Part model, mm, in its own coordinate system. A direction names the side the tool comes from. Coordinates: 2 decimals unless noted, no trailing zeros. Loops run counter-clockwise (first coordinate to the right, second up) from the corner with the lowest first, then second, coordinate; pieces in that order, holes last. Notation, with made-up numbers: M -23.75,-32 L 0.25,-32 A26 cw 0.25,-11 Z; hole C 44.5,17.5 d3. An arc over 180 degrees is marked long. Answer as CSV lines item,"result". Start each with the question number.
Autodesk Inventor part; units mm, degrees
ref_plane "YZ Plane" through (0, 0, 0) normal (1, 0, 0) x (0, 1, 0)
ref_plane "XZ Plane" through (0, 0, 0) normal (0, 1, 0) x (-1, 0, 0)
ref_plane "XY Plane" through (0, 0, 0) normal (0, 0, 1) x (1, 0, 0)
sketch "Sketch1" plane through (0, 0, 0) normal (0, 0, 1) x (1, 0, 0)
  line L0 (0, 0) -> (1800, 0)
  line L1 (0, 0) -> (0, -40)
  line L2 (0, -40) -> (1800, -40)
  line L3 (1800, -40) -> (1800, 0)
  dimension "d0" = 1800
  dimension "d1" = 40
extrude "Extrusion1" add sketch "Sketch1" along normal blind 40
sketch "Sketch2" plane through (0, 0, 40) normal (0, 0, 1) x (1, 0, 0)
  line L0 (0, 0) -> (0, -40)
  line L1 (1800, 0) -> (0, 0)
  line L2 (0, 0) -> (40, 0)
  line L3 (0, -40) -> (1800, -40)
  line L4 (40, -40) -> (0, -40)
  line L5 (0, -40) -> (0, 0)
  line L6 (40, 0) -> (40, -40)
  line L7 (1800, -40) -> (1800, 0)
  line L8 (1800, 0) -> (1760, 0)
  line L9 (1760, -40) -> (1800, -40)
  line L10 (1760, 0) -> (1760, -40)
  line L11 (1800, 0) -> (1800, -40)
  dimension "d5" = 40
  dimension "d6" = 40
extrude "Extrusion2" add sketch "Sketch2" along normal blind 960 contours L1 L6 L3 L0 | L1 L7 L3 L10
sketch "Sketch4" plane through (1760, -40, 40) normal (-1, 0, 0) x (0, 0, 1)
  line L0 (960, 40) -> (960, 0)
  line L1 (960, 40) -> (920, 40)
  line L2 (0, 40) -> (960, 40)
  line L3 (0, 0) -> (960, 0)
  line L4 (920, 0) -> (920, 40)
  line L5 (920, 0) -> (960, 0)
  line L6 (960, 0) -> (960, 40)
  point P0 (-40, 40)
  dimension "d9" = 40
extrude "Extrusion3" add sketch "Sketch4" along normal up to surface (1720 mm away)
sketch "Sketch5" plane through (0, -40, 0) normal (0, -1, 0) x (1, 0, 0)
  line L0 (40, 40) -> (40, 960)
  line L1 (40, 960) -> (40, 1000)
  line L2 (1800, 1000) -> (0, 1000)
  line L3 (0, 1000) -> (0, 960)
  line L4 (0, 0) -> (0, 1000)
  line L5 (40, 960) -> (0, 960)
  line L6 (0, 1000) -> (40, 1000)
  line L7 (1760, 40) -> (1760, 960)
  line L8 (1760, 960) -> (1800, 960)
  line L9 (1800, 0) -> (1800, 1000)
  line L10 (1760, 960) -> (1760, 1000)
  line L11 (1760, 1000) -> (1800, 1000)
  line L12 (1800, 1000) -> (1800, 960)
  line L13 (1760, 40) -> (40, 40)
  line L14 (1760, 40) -> (1800, 40)
  line L15 (1800, 40) -> (1800, 0)
  line L16 (1800, 0) -> (1760, 0)
  line L17 (1800, 0) -> (0, 0)
  line L18 (1760, 0) -> (1760, 40)
  line L19 (0, 40) -> (40, 40)
  line L20 (40, 0) -> (40, 40)
  line L21 (0, 40) -> (0, 0)
  line L22 (40, 0) -> (0, 0)
extrude "Extrusion4" add sketch "Sketch5" along normal blind 710 contours L20 L17 L4 L19 | L5 L3 L2 L1 | L14 L9 L16 L18 | L10 L2 L9 L8
sketch "Sketch6" plane through (1760, -40, 0) normal (-1, 0, 0) x (0, 0, 1)
  line L0 (0, 40) -> (0, -710)
  line L1 (0, -610) -> (40, -610)
  line L2 (40, 0) -> (40, -710)
  line L3 (0, -610) -> (0, -650)
  line L4 (0, -650) -> (40, -650)
  line L5 (40, -650) -> (40, -610)
  line L6 (0, 0) -> (40, 0)
  line L7 (960, 0) -> (960, -710)
  line L8 (960, -610) -> (1000, -610)
  line L9 (1000, 0) -> (1000, -710)
  line L10 (960, -650) -> (1000, -650)
  line L11 (1000, -650) -> (1000, -610)
  line L12 (960, -610) -> (960, -650)
  dimension "d14" = 40
  dimension "d15" = 650
extrude "Extrusion5" add sketch "Sketch6" along normal up to surface (1720 mm away) contours L1 L2 L4 L0 | L8 L9 L10 L7
sketch "Sketch7" plane through (0, -750, 40) normal (0, 0, 1) x (1, 0, 0)
  line L0 (40, 710) -> (40, 100)
  line L1 (40, 100) -> (0, 100)
  line L2 (0, 100) -> (0, 60)
  line L3 (40, 60) -> (40, 0)
  line L4 (0, 60) -> (40, 60)
  line L5 (40, 60) -> (40, 100)
  line L6 (1760, 60) -> (1760, 0)
  line L7 (1760, 60) -> (1800, 60)
  line L8 (1800, 710) -> (1800, 0)
  line L9 (1760, 710) -> (1760, 100)
  line L10 (1800, 100) -> (1760, 100)
  line L11 (1760, 100) -> (1760, 60)
  line L12 (0, 100) -> (0, 60)
  line L13 (0, 710) -> (0, 0)
  line L14 (1800, 100) -> (1800, 60)
  line L15 (0, 100) -> (0, 60)
  point P0 (0, 750)
extrude "Extrusion6" add sketch "Sketch7" along normal up to surface (920 mm away)
sketch "Sketch8" plane through (0, 0, 0) normal (-1, 0, 0) x (0, 0, 1)
  line L0 (40, -650) -> (960, -650)
  line L1 (902, -650) -> (902, -420)
  line L2 (902, -420) -> (722, -420)
  line L3 (722, -420) -> (722, -650)
  line L4 (960, -40) -> (960, -650)
  line L5 (722, -450) -> (902, -450)
  line L6 (722, -650) -> (902, -650)
  line L7 (764.1942, -450) -> (764.1942, -650)
  line L8 (794.1942, -450) -> (794.1942, -650)
  line L9 (826.1942, -450) -> (826.1942, -650)
  line L10 (856.1942, -450) -> (856.1942, -650)
  line L11 (872.1942, -450) -> (872.1942, -650)
  line L12 (748.1942, -450) -> (748.1942, -650)
  point P0 (0, 0)
  dimension "d20" = 230
  dimension "d21" = 58
  dimension "d22" = 180
  dimension "d23" = 30
  dimension "d24" = 30
  dimension "d25" = 30
  dimension "d26" = 32
  dimension "d27" = 16
  dimension "d28" = 16
extrude "Extrusion7" add sketch "Sketch8" against normal blind 30 contours L3 L5 L12 L0 | L3 L2 L1 L5 | L7 L5 L8 L0 | L9 L5 L10 L0 | L1 L0 L11 L5
sketch "Sketch9" plane through (1760, -690, 960) normal (0, 0, -1) x (-1, 0, 0)
  line L0 (0, 40) -> (1720, 40)
  line L1 (110, 40) -> (140, 40)
  line L2 (140, 40) -> (140, 10)
  line L3 (140, 10) -> (110, 10)
  line L4 (110, 10) -> (110, 40)
  line L5 (610, 40) -> (640, 40)
  line L6 (640, 40) -> (640, 10)
  line L7 (640, 10) -> (610, 10)
  line L8 (610, 10) -> (610, 40)
  line L9 (1080, 40) -> (1110, 40)
  line L10 (1110, 40) -> (1110, 10)
  line L11 (1110, 10) -> (1080, 10)
  line L12 (1080, 10) -> (1080, 40)
  line L13 (1580, 40) -> (1610, 40)
  line L14 (1610, 40) -> (1610, 10)
  line L15 (1610, 10) -> (1580, 10)
  line L16 (1580, 10) -> (1580, 40)
  line L17 (-40, -60) -> (-40, 690)
  line L18 (1760, 690) -> (1760, -60)
  point P0 (1610, 40)
  point P1 (1580, 40)
  point P2 (640, 40)
  point P3 (610, 40)
  dimension "d31" = 30
  dimension "d32" = 30
  dimension "d33" = 30
  dimension "d34" = 30
  dimension "d35" = 30
  dimension "d36" = 30
  dimension "d37" = 30
  dimension "d38" = 30
  dimension "d39" = 150
  dimension "d40" = 150
  dimension "d41" = 470
  dimension "d42" = 470
extrude "Extrusion8" add sketch "Sketch9" along normal up to surface (920 mm away)
sketch "Sketch24" plane through (0, -750, 0) normal (0, -1, 0) x (1, 0, 0)
  circle A0 centre (20, 20) radius 6
  line L0 (40, 40) -> (0, 40)
  line L1 (0, 40) -> (0, 0)
  point P0 (0, 20)
  dimension "d95" = 20
  dimension "d96" = 20
  dimension "d97" = 12
sketch "Sketch25" plane through (0, -750, 0) normal (0, -1, 0) x (1, 0, 0)
  circle A0 centre (20, 980) radius 6
  line L0 (40, 1000) -> (0, 1000)
  line L1 (0, 1000) -> (0, 960)
  circle A1 centre (1780, 980) radius 6
  circle A2 centre (1780, 20) radius 6
  line L2 (1760, 0) -> (1800, 0)
  line L3 (1800, 0) -> (1800, 40)
  point P0 (0, 0)
  dimension "d98" = 20
  dimension "d99" = 20
  dimension "d100" = 12
  dimension "d101" = 20
  dimension "d102" = 20
  dimension "d103" = 12
hole "Hole1" at (20, -750, 20) direction (0, 1, 0) diameter 12 depth 20 tip angle 118
hole "Hole2" at (20, -750, 980) at (1780, -750, 980) at (1780, -750, 20) direction (0, 1, 0) diameter 12 depth 20 tip angle 118
properties part number "BangTai"
Q1. Wall check: L1, parallel to Z at x = 20, y = -738.25; L2, parallel to X at y = -741, z = 20; L3, parallel to X at y = -38.5, z = 334.5. Give the ranges that are in metal, low to high.
Q2. Two-plate mould, pull along Z, no slides. Class faces 1 (the face through (888, -670, 40)), 2 (the face through (1780, -720, 960)), 3 (the face through (912, -40, 980)): +Z half, -Z half, draft (parallel to the pull), parting line (faces both ways), or undercut.
Q3. Slice it at A-A, the plane y = -113. Write the cut outline in (x, z).
Q4. Flat gauge pins, fed straight in: P1, Ø9, axis at x = 11, z = 788.5, coming from the +Y side; P2, Ø9, axis at x = 663, z = 334.5, coming from the -Y side; P3, Ø12, axis at x = 1247.5, z = 971, coming from the -Y side; P4, Ø11, axis at x = 20, z = 980, coming from the -Y side. Where does each tip first touch, or does it go through?
Q5. Slice it at B-B, the plane x = 1021.5. Write the cut outline in (y, z).
Q6. Slice it at C-C, the plane z = 923. State how many separate pieces and enclosed holes the cut face has, and give its area (3 significant figures).
Q7. Tool access for faces 4 (the face through (20, -40, 494)), 5 (the face through (1760, -20, 494)), 6 (the face through (40, -341, 20)), 7 (the face through (912, -690, 20)): list every direction of +Z, -Z, +X, -X, +Y, -Y with a clear straight run to the whole face (end or side of a thin tool).
Solved:
1,L1,"z = 0 to 14, 26 to 40, 960 to 974, 986 to 1000"
1,L2,"x = 0 to 14, 26 to 40, 1760 to 1774, 1786 to 1800"
1,L3,"x = 0 to 40, 1760 to 1800"
2,face 1,"undercut"
2,face 2,"undercut"
2,face 3,"draft"
3,outline,"M 0,0 L 40,0 L 40,40 L 0,40 Z; M 0,960 L 40,960 L 40,1000 L 0,1000 Z; M 1760,0 L 1800,0 L 1800,40 L 1760,40 Z; M 1760,960 L 1800,960 L 1800,1000 L 1760,1000 Z"
4,P1,"stops at y = 0"
4,P2,"stops at y = -680"
4,P3,"stops at y = -690"
4,P4,"stops at y = -729.7"
5,outline,"M -690,0 L -650,0 L -650,40 L -690,40 Z; M -690,960 L -650,960 L -650,1000 L -690,1000 Z; M -40,0 L 0,0 L 0,40 L -40,40 Z; M -40,960 L 0,960 L 0,1000 L -40,1000 Z"
6,separate pieces,"8"
6,enclosed holes,"0"
6,area,"10,000 mm2"
7,face 4,"+X, -X"
7,face 5,"+Y, -Y"
7,face 6,"+Z, -Z"
7,face 7,"+Z, -Z, -Y"
